Geometry: final body of the model. Coordinates: model frame, mm. Face numbers are marked on the shaded views. A direction names the side the tool comes from. Coordinates: 2 decimals unless noted, no trailing zeros. Loops run counter-clockwise (first coordinate to the right, second up) from the corner with the lowest first, then second, coordinate; pieces in that order, holes last. Notation, with made-up numbers: (-24, 88) - (9, 88) arc R19 cw to (9, 97) - close; hole circle Ø2 at (64, 80). An arc over 180 degrees is marked (long way). Answer in a Markdown table with one row per item.
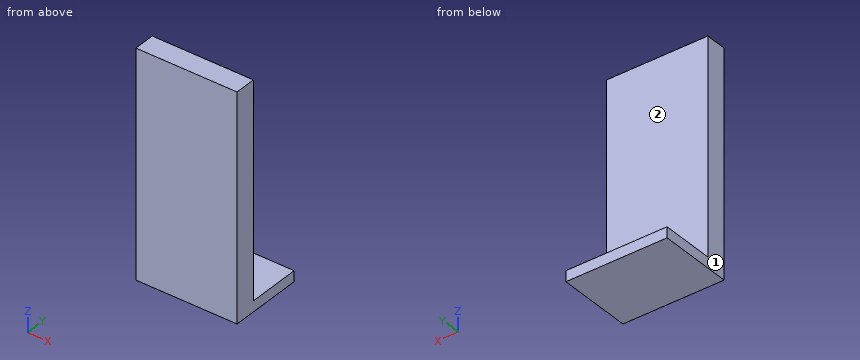
from build123d import *

# Parameters (mm, degrees)
SKETCH1_W           = 950
SKETCH1_H           = 2000
BOSS_EXTRUDE1_DEPTH = 200
SKETCH2_W           = 950
SKETCH2_H           = 100
BOSS_EXTRUDE2_DEPTH = 700


with BuildPart() as part:
    # Sketch1 → Boss-Extrude1 (new body)
    with BuildSketch(Plane(origin=(0, 0, 0), x_dir=(1, 0, 0), z_dir=(0, 1, 0))):
        Rectangle(SKETCH1_W, SKETCH1_H)
    extrude(amount=BOSS_EXTRUDE1_DEPTH)

    # Sketch2 → Boss-Extrude2 (add)
    with BuildSketch(Plane.XZ):
        with Locations((0, -1050)):
            Rectangle(SKETCH2_W, SKETCH2_H)
    extrude(amount=-BOSS_EXTRUDE2_DEPTH)


solid = part.part
(1) Access query for the marked faces 1 and 2. Directions: +Z, -Z, +X, -X, +Y, -Y. A direction counts if a zero-diameter tool reaches every point of the face in a straight line with its end or side. Return the directions, or none.
Verdict:
| item | result |
|---|---|
| face 1 | +Z, -Z, -X, +Y, -Y |
| face 2 | +Z, +X, -X, +Y |
(2) Cut plane C-C on z = -290. Output: boundary loops of the cut face in (x, y).
Verdict:
| item | result |
|---|---|
| outline | (-475, 0) - (475, 0) - (475, 200) - (-475, 200) - close |
(3) First-contact query: pin 1 Ø5 at (x, y) = (271, 299) entering from +Z; pin 2 Ø6 at (x, z) = (-170, -795.5) entering from +Y. Flat tips, straight axial feed; report the tip coordinate or a pass-through.
Verdict:
| item | result |
|---|---|
| pin 1 | stops at z = -1000 |
| pin 2 | stops at y = 200 |
(4) Ray query, probe 1 along Z at (x, y) = (305, 272.5); probe 2 along Y at (x, z) = (129.5, -63). Return the intervals inside material, ascending.
Verdict:
| item | result |
|---|---|
| probe 1 | z = -1100 to -1000 |
| probe 2 | y = 0 to 200 |
(5) Cut plane A-A on x = 328. Output: boundary loops of the cut face in (y, z).
Verdict:
| item | result |
|---|---|
| outline | (0, -1100) - (700, -1100) - (700, -1000) - (200, -1000) - (200, 1000) - (0, 1000) - close |
(6) Cut plane B-B on y = 623.5. Output: boundary loops of the cut face in (x, z).
Verdict:
| item | result |
|---|---|
| outline | (-475, -1100) - (475, -1100) - (475, -1000) - (-475, -1000) - close |
